Check sheet for the modelled part. Datum: model origin and axes. Units: mm. Face numbers are marked on the shaded views. A direction names the side the tool comes from. Round coordinates to 2 decimals unless told otherwise and drop trailing zeros. Loops run counter-clockwise (first coordinate to the right, second up) from the corner with the lowest first, then second, coordinate; pieces in that order, holes last. Notation, with made-up numbers: (-21.75, -37.5) - (22.25, -37.5) arc R20 ccw to (22.25, -12.5) - close; hole circle Ø9 at (12.25, 39). An arc over 180 degrees is marked (long way). Put each result on its own line as item: value. Start each with the question number.
Item 1: Section check D-D, the plane z = 1.5. Record the cut outline in (x, y), and give its area (3 significant figures).
Item 2: Gauge pin test, flat ends, axial feed: pin 1 Ø10 at (x, z) = (13.5, 14.5) entering from +Y; pin 2 Ø3.5 at (x, z) = (20.5, 6) entering from +Y. Record the tip position at first contact, or that the pin passes through.
Item 3: Draft check along Y on the marked faces 4, 5 and 6. Enter one of: pulls with the +Y half, pulls with the -Y half, needs draft (parallel to the pull), parting line crosses it, or undercut.
Item 4: Section check A-A, the plane z = 10. Record the cut outline in (x, y).
Item 5: Section check C-C, the plane y = -9. Record the cut outline in (x, z).
Item 6: Section check B-B, the plane y = -2. Record the cut outline in (x, z).
Item 7: Tool access check on the marked faces 1, 2 and 3. Record the directions out of +Z, -Z, +X, -X, +Y, -Y that give a thin tool (end or side, any length) a straight path to the whole face; none if there is none.
Item 8: Material ranges on line 1 along Y through (x, z) = (1.3, 10); line 2 along X through (y, z) = (-11.25, 7.5); line 3 along Y through (x, z) = (14, 1.75), recorded low to high.
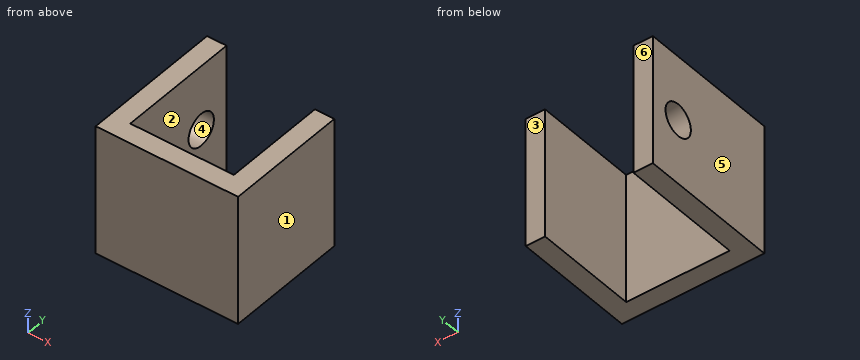
Autodesk Inventor part; units mm, degrees
ref_plane "YZ Plane" through (0, 0, 0) normal (1, 0, 0) x (0, 1, 0)
ref_plane "XZ Plane" through (0, 0, 0) normal (0, 1, 0) x (-1, 0, 0)
ref_plane "XY Plane" through (0, 0, 0) normal (0, 0, 1) x (1, 0, 0)
sketch "Sketch1" plane through (0, 0, 0) normal (0, 0, 1) x (1, 0, 0)
  line L0 (0, 0) -> (22, 0)
  line L1 (22, 0) -> (22, -19)
  line L2 (22, -19) -> (0, -19)
  line L3 (0, -19) -> (0, 0)
  line L4 (3, 0) -> (19, 0)
  line L5 (19, 0) -> (19, -16)
  line L6 (19, -16) -> (3, -16)
  line L7 (3, -16) -> (3, 0)
  dimension "d0" = 22
  dimension "d1" = 19
  dimension "d2" = 3
  dimension "d3" = 3
  dimension "d4" = 3
extrude "Extrusion1" add sketch "Sketch1" along normal blind 20 contours L0 L7 L6 L5 L1 L2 L3
sketch "Sketch2" plane through (0, -19, 0) normal (-1, 0, 0) x (0, 0, 1)
  line L0 (0, 19) -> (20, 19)
  line L1 (0, 19) -> (20, 19)
  line L2 (20, 19) -> (20, 22)
  line L3 (20, 22) -> (0, 22)
  line L4 (0, 22) -> (0, 19)
  dimension "d7" = 3
extrude "Extrusion2" add sketch "Sketch2" against normal blind 3
sketch "Sketch3" plane through (0, -19, 0) normal (-1, 0, 0) x (0, 0, 1)
  line L0 (0, 22) -> (0, 0)
  line L1 (20, 22) -> (0, 22)
  circle A0 centre (10, 17) radius 2.5
  point P0 (0, 19)
  dimension "d10" = 10
  dimension "d11" = 5
  dimension "d12" = 5
extrude "Extrusion3" cut sketch "Sketch3" against normal blind 5
equation "\"d3\" = d2"
equation "\"d4\" = d2"
properties part number "LED strip mount v01"
Check result:
1. outline: (0, -19) - (22, -19) - (22, 0) - (19, 0) - (19, -16) - (3, -16) - (3, 3) - (0, 3) - close
1. area: 171 mm²
2. pin 1: y = -16
2. pin 2: y = 0
3. face 4: undercut
3. face 5: needs draft
3. face 6: pulls with the +Y half
4. outline: (0, -19) - (22, -19) - (22, 0) - (19, 0) - (19, -16) - (3, -16) - (3, -4.5) - (0, -4.5) - close; (0, 0.5) - (3, 0.5) - (3, 3) - (0, 3) - close
5. outline: (0, 0) - (3, 0) - (3, 20) - (0, 20) - close; (19, 0) - (22, 0) - (22, 20) - (19, 20) - close
6. outline: (0, 0) - (3, 0) - (3, 7.5) - (0, 7.5) - close; (0, 12.5) - (3, 12.5) - (3, 20) - (0, 20) - close; (19, 0) - (22, 0) - (22, 20) - (19, 20) - close
7. face 1: +Z, -Z, +X, +Y, -Y
7. face 2: +Z, -Z, +Y
7. face 3: +Z, -Z, +X, +Y
8. line 1: -19 to -4.5, 0.5 to 3
8. line 2: 0 to 3, 19 to 22
8. line 3: -19 to -16
